The model under review builds one solid part; all positions refer to its coordinate system, in mm. Round coordinates to 2 decimals unless told otherwise and drop trailing zeros. Order: outer loops, then holes, each group sorted by start corner. A loop starts at its lowest first (then second) coordinate and runs counter-clockwise, first axis right, second up.
```python
from build123d import *

# Parameters (mm, degrees)
SKETCH_1_R               = 4
SKETCH_1_R_2             = 1.25
EXTRUDE_1_DEPTH          = 10
M4X0_7_1_D               = 3.3
M4X0_7_1_DEPTH           = 11.5
M4X0_7_1_TIP             = 0.991420021
M4X0_7_1_ON_FACE_2_D     = 3.3
M4X0_7_1_ON_FACE_2_DEPTH = 11.5
M4X0_7_1_ON_FACE_2_TIP   = 0.991420021
M4X0_7_1_ON_FACE_3_D     = 3.3
M4X0_7_1_ON_FACE_3_DEPTH = 11.5
M4X0_7_1_ON_FACE_3_TIP   = 0.991420021


with BuildPart() as part:
    # ｽｹｯﾁ1 → ﾎﾞｽ - 押し出し1 (new body, symmetric)
    with BuildSketch(Plane.XY):
        Circle(SKETCH_1_R)
        Circle(SKETCH_1_R_2, mode=Mode.SUBTRACT)
        Circle(SKETCH_1_R_2)
    extrude(amount=EXTRUDE_1_DEPTH, both=True)

    # M4x0.7 ねじ穴1
    with Locations(Plane(origin=(0, 0, -10), x_dir=(0, -1, 0), z_dir=(0, 0, -1))):
        with Locations((0, 0)):
            Hole(M4X0_7_1_D / 2, depth=M4X0_7_1_DEPTH)
            with Locations((0, 0, -(M4X0_7_1_DEPTH + M4X0_7_1_TIP / 2))):  # 118° drill point
                Cone(0, M4X0_7_1_D / 2, M4X0_7_1_TIP, mode=Mode.SUBTRACT)

    # M4x0.7 ねじ穴1 on face 2
    with Locations(Plane(origin=(0, 0, 0), x_dir=(0, -1, 0), z_dir=(0, 0, -1))):
        with Locations((0, 0), (-3.399491027, 15.650266716), (-2.590821191, 13.66210105)):
            Hole(M4X0_7_1_ON_FACE_2_D / 2, depth=M4X0_7_1_ON_FACE_2_DEPTH)
            with Locations((0, 0, -(M4X0_7_1_ON_FACE_2_DEPTH + M4X0_7_1_ON_FACE_2_TIP / 2))):  # 118° drill point
                Cone(0, M4X0_7_1_ON_FACE_2_D / 2, M4X0_7_1_ON_FACE_2_TIP, mode=Mode.SUBTRACT)

    # M4x0.7 ねじ穴1 on face 3
    with Locations(Plane.XY.offset(10)):
        with Locations((0, 0)):
            Hole(M4X0_7_1_ON_FACE_3_D / 2, depth=M4X0_7_1_ON_FACE_3_DEPTH)
            with Locations((0, 0, -(M4X0_7_1_ON_FACE_3_DEPTH + M4X0_7_1_ON_FACE_3_TIP / 2))):  # 118° drill point
                Cone(0, M4X0_7_1_ON_FACE_3_D / 2, M4X0_7_1_ON_FACE_3_TIP, mode=Mode.SUBTRACT)


solid = part.part
```
(1) Draft analysis for pull direction Y (two halves, no side actions). For faces 1 (the cylindrical face through (-0.867, -3.905, 0.14)), 2 (the flat face through (2, 0, 10)), 3 (the cylindrical face through (-1.115, -1.216, 0.14)), state which applies: pulls with the +Y half, pulls with the -Y half, needs draft (parallel to the pull), parting line crosses it, or undercut.
Data:
face 1: parting line crosses it
face 2: needs draft
face 3: undercut
(2) Consider section C-C (z = 5.75). Write out the cut boundary in (x, y), and give its area (3 significant figures).
Data:
outline: circle Ø8 at (0, 0); hole circle Ø3.3 at (0, 0)
area: 41.7 mm2
(3) Insertion check: pin 1 (1 mm diameter, centred on x = 1, z = 4.5, fed in from +Y); pin 2 (3 mm diameter, centred on x = 0, y = 0, fed in from +Z). Each pin has a flat end and moves straight along its axis. Give the tip position at first contact, or say it passes through.
Data:
pin 1: stops at y = 3.97
pin 2: passes through
(4) Consider section D-D (x = 3). Write out the cut boundary in (y, z).
Data:
outline: (-2.65, -10) - (2.65, -10) - (2.65, 10) - (-2.65, 10) - close
(5) To check wall thickness, follow probe 1 along X at (y, z) = (-0.25, -1); probe 2 along X at (y, z) = (0.75, 9); probe 3 along Y at (x, z) = (-1.5, -7.75). State the ranges of each line that lie inside material, in increasing order.
Data:
probe 1: x = -3.99 to -1.63, 1.63 to 3.99
probe 2: x = -3.93 to -1.47, 1.47 to 3.93
probe 3: y = -3.71 to -0.69, 0.69 to 3.71
(6) Consider section A-A (y = 0). Write out the cut boundary in (x, z), and give its area (3 significant figures).
Data:
outline: (-4, -10) - (-1.65, -10) - (-1.65, 10) - (-4, 10) - close; (1.65, -10) - (4, -10) - (4, 10) - (1.65, 10) - close
area: 94.0 mm2
